Autodesk Inventor part; units mm, degrees
ref_plane "YZ Plane" through (0, 0, 0) normal (1, 0, 0) x (0, 1, 0)
ref_plane "XZ Plane" through (0, 0, 0) normal (0, 1, 0) x (-1, 0, 0)
ref_plane "XY Plane" through (0, 0, 0) normal (0, 0, 1) x (1, 0, 0)
sketch "Sketch1" plane through (0, 0, 0) normal (0, 0, 1) x (1, 0, 0)
  line L0 (-22.4, 0) -> (22.4, 0) construction
  line L1 (0, -22.4) -> (0, 22.4) construction
  line L2 (-16, 16) -> (16, 16)
  line L3 (16, 16) -> (16, -16)
  line L4 (16, -16) -> (-16, -16)
  line L5 (-16, -16) -> (-16, 16)
  line L6 (8, 16) -> (-16, 8)
  line L7 (-16, -8) -> (8, -16)
  line L8 (16, 8) -> (8, 8)
  line L9 (8, 8) -> (8, -8)
  line L10 (8, -8) -> (16, -8)
  point P0 (-16, 0)
  point P1 (0, 16)
  point P2 (8, 0)
  dimension "d0" = 32
  dimension "d1" = 32
  dimension "d5" = 16
  dimension "d9" = 8
  dimension "d10" = 16
extrude "Extrusion1" add sketch "Sketch1" along normal blind 9.6 contours L2 L3 L8 L9 L10 L4 L7 L5 L6 | L3 L10 L9 L8
sketch "Sketch2" plane through (0, 0, 0) normal (0, 1, 0) x (-1, 0, 0)
  line L0 (-16, 0) -> (-16, 9.6)
  line L1 (-16, 9.6) -> (-8, 9.6)
  line L2 (16, 0) -> (16, 9.6)
  line L3 (16, 0) -> (-16, 0)
  line L4 (-8, 9.6) -> (16, 1.6)
  dimension "d6" = 1.6
extrude "Extrusion2" cut sketch "Sketch2" along normal through all both and the other way through all keep common part
extrude "Extrusion4" cut sketch "Sketch1" along normal through all both and the other way through all contours L3 L10 L9 L8
shell "Shell1" thickness 0.8 removed faces 1 at (-8, 2.6667, 0)
sketch "Sketch3" plane through (0, 0, 9.6) normal (0, 0, 1) x (1, 0, 0)
  line L0 (16, 16) -> (16, -16) construction
  line L1 (-22.4, 0) -> (22.4, 0) construction
  line L2 (12, 12) -> (12, -12) construction
  circle A0 centre (12, 12) radius 2.5
  circle A1 centre (12, -12) radius 2.5
  point P0 (12, 0)
  dimension "d11" = 4
  dimension "d12" = 24
  dimension "d13" = 5
extrude "Extrusion3" add sketch "Sketch3" along normal blind 1.6
properties part number "LEGO Brick 4858" material "Steel"
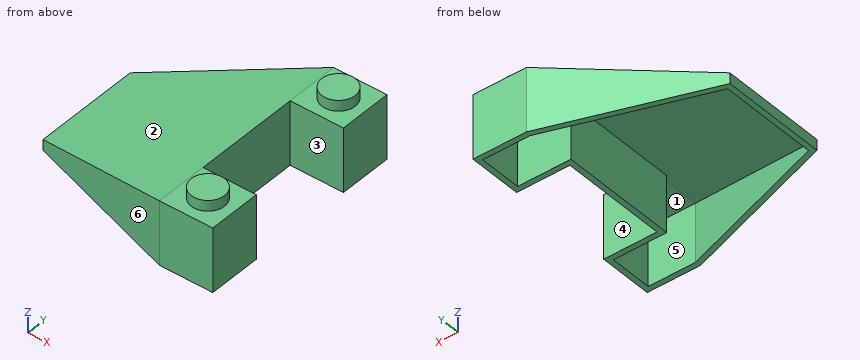
Work out the finished part from the listing and answer in its coordinate system (mm). Face numbers are marked on the shaded views. A direction names the side the tool comes from. Give positions to 0.01 mm unless a question says otherwise; leave off trailing zeros. Loops run counter-clockwise (first coordinate to the right, second up) from the corner with the lowest first, then second, coordinate; pieces in that order, holes last. Notation, with made-up numbers: (-21.5, 46.25) - (16.5, 46.25) arc R25 ccw to (16.5, 59.25) - close; hole circle Ø4 at (43, 24). An arc over 180 degrees is marked (long way). One line per question, with ' | ' between items.
(1) The part is cut by section B-B (y = 3). Write down the section's boundary in (x, z).
Recorded:
outline: (-16, 0) - (-15.2, 0) - (-15.2, 1.02) - (7.2, 8.49) - (7.2, 0) - (8, 0) - (8, 9.6) - (-16, 1.6) - close
(2) A tool of negligible diameter and unlimited length cuts with its end or side. For the marked faces 4, 5 and 6, from which of +Z, -Z, +X, -X, +Y, -Y can it reach the whole face along a straight path? Write none if from no direction.
Recorded:
face 4: +Z, -Z, +X | face 5: -Z | face 6: +Z, -Z, -X, -Y
(3) The part is cut by section A-A (x = 12). Write down the section's boundary in (y, z), then the cut area to 3 significant figures.
Recorded:
outline: (-16, 0) - (-15.2, 0) - (-15.2, 8.8) - (-8.8, 8.8) - (-8.8, 0) - (-8, 0) - (-8, 9.6) - (-9.5, 9.6) - (-9.5, 11.2) - (-14.5, 11.2) - (-14.5, 9.6) - (-16, 9.6) - close; (8, 0) - (8.8, 0) - (8.8, 8.8) - (15.2, 8.8) - (15.2, 0) - (16, 0) - (16, 9.6) - (14.5, 9.6) - (14.5, 11.2) - (9.5, 11.2) - (9.5, 9.6) - (8, 9.6) - close | area: 57.0 mm²
(4) The part is cut by section D-D (x = -12). Write down the section's boundary in (y, z).
Recorded:
outline: (-9.33, 0) - (-8.49, 0) - (-8.49, 2.09) - (8.49, 2.09) - (8.49, 0) - (9.33, 0) - (9.33, 2.93) - (-9.33, 2.93) - close
(5) Each of these flat-tipped pins is pushed along its axis until it touches: pin 1 Ø6 at (x, y) = (-8.5, 7.5) entering from +Z; pin 2 Ø1.1 at (y, z) = (1.5, 0.5) entering from +X; pin 3 Ø6 at (x, z) = (2, 3) entering from -Y. Where does it stop, or does it pass through?
Recorded:
pin 1: stops at z = 5.1 | pin 2: stops at x = 8 | pin 3: stops at y = -15
(6) Straight lines are drawn through the part: probe 1 along Y at (x, z) = (9.5, 7.75); probe 2 along X at (y, z) = (5.5, 1); probe 3 along Y at (x, z) = (5.5, 5.5). For each, find the intervals that lie inside material, in ascending order.
Recorded:
probe 1: y = -16 to -15.2, -8.8 to -8, 8 to 8.8, 15.2 to 16 | probe 2: x = -16 to -15.2, 7.2 to 8 | probe 3: y = -15.17 to -14.32, 14.32 to 15.17
(7) The mould has two halves that part along X. Classify the marked faces 1, 2 and 3: +X half, -X half, draft (parallel to the pull), parting line (faces both ways), or undercut.
Recorded:
face 1: undercut | face 2: -X half | face 3: draft
(8) The part is cut by section C-C (z = 4). Write down the section's boundary in (x, y).
Recorded:
outline: (-8.8, -10.4) - (8, -16) - (16, -16) - (16, -8) - (8, -8) - (8, 8) - (16, 8) - (16, 16) - (8, 16) - (-8.8, 10.4) - close; hole (-6.27, -10.4) - (8.13, -15.2) - (15.2, -15.2) - (15.2, -8.8) - (7.2, -8.8) - (7.2, 8.8) - (15.2, 8.8) - (15.2, 15.2) - (8.13, 15.2) - (-6.27, 10.4) - close
